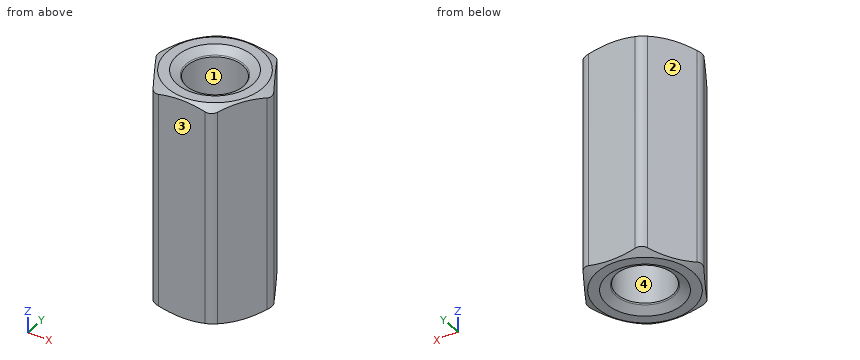
```python
from build123d import *

# Parameters (mm, degrees)
SKETCH4_R           = 1.75
BOSS_EXTRUDE1_DEPTH = 5
SKETCH5_OUTSIDE_W   = 49.716
SKETCH5_OUTSIDE_H   = 49.02
SKETCH5_OUTSIDE_R   = 2.1375
CUT_EXTRUDE1_DEPTH  = 11.574142991
CUT_EXTRUDE1_DRAFT  = -60
SKETCH6_OUTSIDE_W   = 49.716
SKETCH6_OUTSIDE_H   = 49.02
SKETCH6_OUTSIDE_R   = 2.1375
CUT_EXTRUDE2_DEPTH  = 11.574142991
CUT_EXTRUDE2_DRAFT  = -60
FILLET1_R           = 0.45
BOSS_EXTRUDE2_START = -5
SKETCH7_R           = 1.69375
BOSS_EXTRUDE2_DEPTH = 4.8
SKETCH8_W           = 4.8
SKETCH8_H           = 1.25
CIRPATTERN1_COUNT   = 2


with BuildPart() as part:
    # Sketch3 → Revolve1 (revolve)
    with BuildSketch(Plane(origin=(0, 0, 0), x_dir=(0, 0, -1), z_dir=(1, 0, 0))):
        Polygon((-4.743800818, 1.25), (-0.2, 1.25), (-0.2, 0), (0.2, 0), (0.2, 1.25), (4.743800818, 1.25), (5, 1.69375), (5, 2.25), (0, 2.25), (-5, 2.25), (-5, 1.69375), align=None)
        Polygon((-4.743800818, 1.25), (-0.2, 1.25), (-0.2, 0), (0.2, 0), (0.2, 1.25), (4.743800818, 1.25), (5, 1.69375), (5, 2.25), (0, 2.25), (-5, 2.25), (-5, 1.69375), align=None)
    revolve(axis=Axis((0, 0, 0.2), (0, 0, 1)))

    # Sketch4 → Boss-Extrude1 (add, symmetric)
    with BuildSketch(Plane.XY):
        Polygon((-1.299038106, 2.25), (-2.598076211, 0), (-1.299038106, -2.25), (1.299038106, -2.25), (2.598076211, 0), (1.299038106, 2.25), align=None)
        Circle(SKETCH4_R, mode=Mode.SUBTRACT)
    extrude(amount=BOSS_EXTRUDE1_DEPTH, both=True)


with BuildPart() as cut_extrude1_tool:
    # Sketch5 outside → Cut-Extrude1 (with draft: the straight prism first)
    with BuildSketch(Plane.XY.offset(5)):
        Rectangle(SKETCH5_OUTSIDE_W, SKETCH5_OUTSIDE_H)
        Circle(SKETCH5_OUTSIDE_R, mode=Mode.SUBTRACT)
    extrude(amount=-CUT_EXTRUDE1_DEPTH)
    # Cut-Extrude1: the draft: its side faces are tilted about the plane it starts from
    cut_extrude1_sides = [cut_extrude1_tool.faces().sort_by_distance(p)[0] for p in [
        (0, -24.51, -0.787071496),
        (24.858, 0, -0.787071496),
        (0, 24.51, -0.787071496),
        (-24.858, 0, -0.787071496),
        (-2.1375, 0, -0.787071496),
    ]]
    draft(cut_extrude1_sides, Plane.XY.offset(5), CUT_EXTRUDE1_DRAFT)


with BuildPart() as part_1:
    add(part.part)

    # Cut-Extrude1: cut by cut_extrude1_tool
    add(cut_extrude1_tool.part, mode=Mode.SUBTRACT)


with BuildPart() as cut_extrude2_tool:
    # Sketch6 outside → Cut-Extrude2 (with draft: the straight prism first)
    with BuildSketch(Plane(origin=(0, 0, -5), x_dir=(-1, 0, 0), z_dir=(0, 0, -1))):
        Rectangle(SKETCH6_OUTSIDE_W, SKETCH6_OUTSIDE_H)
        Circle(SKETCH6_OUTSIDE_R, mode=Mode.SUBTRACT)
    extrude(amount=-CUT_EXTRUDE2_DEPTH)
    # Cut-Extrude2: the draft: its side faces are tilted about the plane it starts from
    cut_extrude2_sides = [cut_extrude2_tool.faces().sort_by_distance(p)[0] for p in [
        (0, -24.51, 0.787071496),
        (-24.858, 0, 0.787071496),
        (0, 24.51, 0.787071496),
        (24.858, 0, 0.787071496),
        (2.1375, 0, 0.787071496),
    ]]
    draft(cut_extrude2_sides, Plane(origin=(0, 0, -5), x_dir=(-1, 0, 0), z_dir=(0, 0, -1)), CUT_EXTRUDE2_DRAFT)


with BuildPart() as part_2:
    add(part_1.part)

    # Cut-Extrude2: cut by cut_extrude2_tool
    add(cut_extrude2_tool.part, mode=Mode.SUBTRACT)

    # Fillet1
    # the kernel refuses this fillet: 0.45 mm, written as the material it takes off along each edge
    with BuildSketch(Plane(origin=(1.299038106, 2.25, 5.383605253), x_dir=(-1, 0, 0), z_dir=(0, 0, -1)), Plane(origin=(-1.299038106, 2.25, 5.383605253), x_dir=(-0.49999999999999967, -0.8660254037844387, 0), z_dir=(0, 0, -1))) as fillet1_piece_1:
        with BuildLine():
            CenterArc((FILLET1_R * 0.57735026919, -FILLET1_R), FILLET1_R, 90, 60)
            Line((-FILLET1_R * 0.288675134595, -FILLET1_R * 0.5), (0, 0))
            Line((0, 0), (FILLET1_R * 0.57735026919, 0))
        make_face()
    extrude(amount=10.767210506, mode=Mode.SUBTRACT)
    with BuildSketch(Plane(origin=(-2.598076211, 0, -5.383605253), x_dir=(0.5000000000000006, -0.8660254037844384, 0), z_dir=(0, 0, 1)), Plane(origin=(-1.299038106, -2.25, -5.383605253), x_dir=(1, 0, 0), z_dir=(0, 0, 1)), Plane(origin=(1.299038106, -2.25, -5.383605253), x_dir=(0.49999999999999967, 0.8660254037844387, 0), z_dir=(0, 0, 1)), Plane(origin=(2.598076211, 0, 5.383605253), x_dir=(-0.5, -0.8660254037844388, 0), z_dir=(0, 0, -1))) as fillet1_piece_2:
        with BuildLine():
            CenterArc((FILLET1_R * 0.57735026919, FILLET1_R), FILLET1_R, 210, 60)
            Line((-FILLET1_R * 0.288675134595, FILLET1_R * 0.5), (0, 0))
            Line((0, 0), (FILLET1_R * 0.57735026919, 0))
        make_face()
    extrude(amount=10.767210506, mode=Mode.SUBTRACT)

    # Sketch7 → Boss-Extrude2 (add)
    with BuildSketch(Plane(origin=(0, 0, 0), x_dir=(-1, 0, 0), z_dir=(0, 0, -1)).offset(BOSS_EXTRUDE2_START)):
        Circle(SKETCH7_R)
    extrude(amount=BOSS_EXTRUDE2_DEPTH)

    # SurfaceCut1
    split(bisect_by=Plane.XY, keep=Keep.TOP)


with BuildPart() as body_2:
    # Sketch8 → Revolve2 (revolve)
    with BuildSketch(Plane(origin=(0, 0, 0), x_dir=(0, 0, -1), z_dir=(1, 0, 0))):
        with Locations((-2.6, 0.625)):
            Rectangle(SKETCH8_W, SKETCH8_H)
    revolve(axis=Axis((0, 0, 0.2), (0, 0, 1)))


with BuildPart() as part_3:
    add(part_2.part)

    # Combine1: cut body 2
    add(body_2.part, mode=Mode.SUBTRACT)

    # Cut-Extrude3 cone 1 section (through the dimple's axis) → Cut-Extrude3 (revolve, cut)
    with BuildSketch(Plane(origin=(0, 0, 5), x_dir=(0, -1, 0), z_dir=(1, 0, 0))):
        Polygon((0, 0), (1.69375, 0), (0, 0.977887018), align=None)
    revolve(axis=Axis((0, 0, 5), (0, 0, -1)), mode=Mode.SUBTRACT)

    # Cut-Extrude4 cone 1 section (through the dimple's axis) → Cut-Extrude4 (revolve, cut)
    with BuildSketch(Plane(origin=(0, 0, 4.768157783), x_dir=(0, -1, 0), z_dir=(1, 0, 0))):
        Polygon((0, 0), (1.3008, 0), (0, 1.3008), align=None)
    revolve(axis=Axis((0, 0, 4.768157783), (0, 0, -1)), mode=Mode.SUBTRACT)


with BuildPart() as cirpattern1_1:
    # CirPattern1: pattern copy
    add(part_3.part.rotate(Axis((0, 0, 0), (1, 0, 0)), 1 * 360 / CIRPATTERN1_COUNT))


with BuildPart() as part_4:
    add(part_3.part)

    # Combine2: union CirPattern1_1
    add(cirpattern1_1.part)


solid = part_4.part
```
Input: part model. Units: mm. Frame: model coordinates. Face numbers are marked on the shaded views. Round coordinates to 2 decimals unless told otherwise and drop trailing zeros. Write each loop counter-clockwise with the first axis right and the second up, starting at its lowest first coordinate (ties: lowest second). Pieces come first, ordered by that corner, then holes. Notation, with made-up numbers: (53, -39) - (105, -39) arc R25 cw to (105, -15) - close; hole circle Ø5 at (57, 0). An arc over 180 degrees is marked (long way). Write item = value, one per line.
(1) Pull-direction query (Y, two-part tool) for the marked faces 1, 2, 3 and 4; classes: +Y half, -Y half, draft (parallel to the pull), parting line (faces both ways), or undercut.
Geometry check:
face_1 = undercut
face_2 = +Y half
face_3 = -Y half
face_4 = undercut
(2) Material intervals for probe 1 along X at (y, z) = (0, -2.35); probe 2 along Y at (x, z) = (0, 2.35); probe 3 along Y at (x, z) = (2, 2.25), sorted ascending.
Geometry check:
probe_1 = -2.53 to -1.25, 1.25 to 2.53
probe_2 = -2.25 to -1.25, 1.25 to 2.25
probe_3 = -1.04 to 1.04
(3) Contact query for flat-ended pins moving along their axis: pin 1 Ø1.5 at (x, y) = (0, 0) entering from +Z; pin 2 Ø0.8 at (x, y) = (0, 0.5) entering from -Z. Output: stop coordinate, or through.
Geometry check:
pin_1 = 0.2
pin_2 = -0.2
(4) Section query A-A on z = 0.75. Output: boundary loops of the cut face in (x, y) (3 decimals), then the cut area to 3 significant figures.
Geometry check:
outline = (-2.468, -0.225) - (-1.429, -2.025) arc R0.45 ccw to (-1.039, -2.25) - (1.039, -2.25) arc R0.45 ccw to (1.429, -2.025) - (2.468, -0.225) arc R0.45 ccw to (2.468, 0.225) - (1.429, 2.025) arc R0.45 ccw to (1.039, 2.25) - (-1.039, 2.25) arc R0.45 ccw to (-1.429, 2.025) - (-2.468, 0.225) arc R0.45 ccw to start; hole circle Ø2.5 at (0, 0)
area = 12.6 mm^2
